The listing builds one solid part. Answer for the finished solid, in the listing's coordinates (mm). Face numbers are marked on the shaded views. Coordinates: 2 decimals unless noted, no trailing zeros. Write each loop counter-clockwise with the first axis right and the second up, starting at its lowest first coordinate (ties: lowest second). Pieces come first, ordered by that corner, then holes.
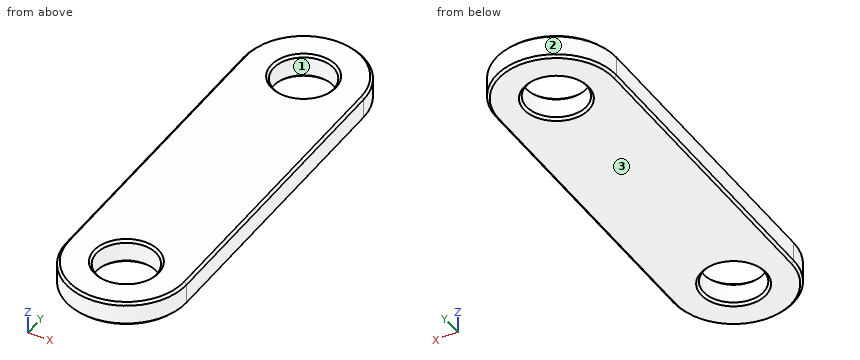
from build123d import *

# Parameters (mm, degrees)
SKETCH2_R           = 25
BOSS_EXTRUDE1_DEPTH = 20
CHAMFER1_SIZE       = 2


with BuildPart() as part:
    # Sketch2 → Boss-Extrude1 (new body)
    with BuildSketch(Plane.XY):
        with BuildLine():
            Line((50, 127.5), (50, -127.5))
            ThreePointArc((50, -127.5), (0, -177.5), (-50, -127.5))
            Line((-50, -127.5), (-50, 127.5))
            ThreePointArc((-50, 127.5), (0, 177.5), (50, 127.5))
        make_face()
        with Locations((0, 127.5)):
            Circle(SKETCH2_R, mode=Mode.SUBTRACT)
        with Locations((0, -127.5)):
            Circle(SKETCH2_R, mode=Mode.SUBTRACT)
    extrude(amount=BOSS_EXTRUDE1_DEPTH)

    # Chamfer1
    chamfer1_edges = [part.edges().sort_by_distance(p)[0] for p in [
        (-25, 127.5, 0),
        (-25, 127.5, 20),
        (0, -177.5, 20),
        (-25, -127.5, 0),
        (-25, -127.5, 20),
        (50, 0, 20),
        (0, 177.5, 20),
        (50, 0, 0),
        (0, -177.5, 0),
        (-50, 0, 0),
        (0, 177.5, 0),
        (-50, 0, 20),
    ]]
    chamfer(chamfer1_edges, length=CHAMFER1_SIZE)


solid = part.part
Q1. The part is cut by section A-A, the plane x = 0. Write down the section's boundary in (y, z).
Answers below:
outline: (-177.5, 2) - (-175.5, 0) - (-154.5, 0) - (-152.5, 2) - (-152.5, 18) - (-154.5, 20) - (-175.5, 20) - (-177.5, 18) - close; (-102.5, 2) - (-100.5, 0) - (100.5, 0) - (102.5, 2) - (102.5, 18) - (100.5, 20) - (-100.5, 20) - (-102.5, 18) - close; (152.5, 2) - (154.5, 0) - (175.5, 0) - (177.5, 2) - (177.5, 18) - (175.5, 20) - (154.5, 20) - (152.5, 18) - close
Q2. Determine the mould class of the marked faces 1, 2 and 3 for opening direction Y: released by +Y, released by -Y, zero draft, split by the parting line, or undercut.
Answers below:
face 1: undercut
face 2: released by +Y
face 3: zero draft
Q3. Given pin 1 (3 mm diameter, centred on x = -9, z = 7.5, fed in from -Y); pin 2 (1 mm diameter, centred on x = 26.5, z = 4.5, fed in from +Y); pin 3 (1 mm diameter, centred on x = -39.5, z = 11, fed in from +Y), each flat-ended and moving along its own axis, determine where each tip first touches the part or whether it passes through.
Answers below:
pin 1: stops at y = -176.93
pin 2: stops at y = 170.21
pin 3: stops at y = 158.79
Q4. The part is cut by section C-C, the plane x = 22. State how many separate pieces and enclosed holes the cut face has, then the cut area to 3 significant figures.
Answers below:
separate pieces: 3
enclosed holes: 0
area: 5,910 mm2
Q5. The part is cut by section B-B, the plane z = 14.75. Write down the section's boundary in (x, y), then the cut area to 3 significant figures.
Answers below:
outline: (-50, -127.5) arc R50 ccw to (50, -127.5) - (50, 127.5) arc R50 ccw to (-50, 127.5) - close; hole circle Ø50 at (0, -127.5); hole circle Ø50 at (0, 127.5)
area: 29,400 mm2
Q6. Find the intervals of material crossed by probe 1 along Y at (x, z) = (0, 8.25); probe 2 along Y at (x, z) = (20, 5.5); probe 3 along X at (y, z) = (-122, 16), in increasing order.
Answers below:
probe 1: y = -177.5 to -152.5, -102.5 to 102.5, 152.5 to 177.5
probe 2: y = -173.33 to -142.5, -112.5 to 112.5, 142.5 to 173.33
probe 3: x = -50 to -24.39, 24.39 to 50
